The figure shows three views and two pictorial views of one solid part (mm, origin at its lowest corner). Answer the questions. A direction names the side the tool comes from. Coordinates: 2 decimals unless noted, no trailing zeros. Order: outer loops, then holes, each group sorted by start corner. A loop starts at its lowest first (then second) coordinate and runs counter-clockwise, first axis right, second up. Notation, with made-up numbers: M 65,-35 L 99,-35 A20 ccw 99,-2 Z; hole C -17,-16 d4. An arc over 180 degrees is marked long. Use a Markdown table: item, result.
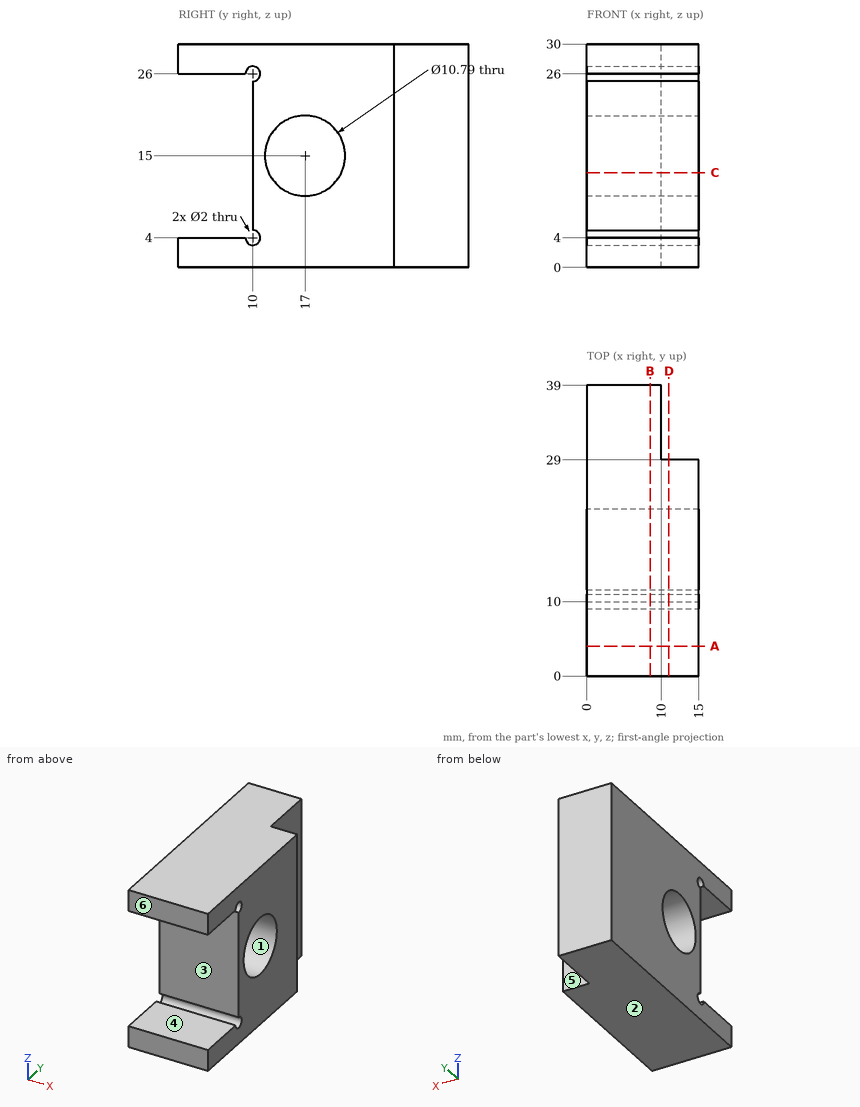
1. Section C-C on z = 12.75 is taken. Determine the outline of the cut face in (x, y).
Answers below:
| item | result |
|---|---|
| outline | M 0,10 L 15,10 L 15,12.1 L 0,12.1 Z; M 0,21.9 L 15,21.9 L 15,29 L 10,29 L 10,39 L 0,39 Z |
2. Find the intervals of material crossed by probe 1 along Z at (x, y) = (4.25, 8.5); probe 2 along Y at (x, z) = (12.5, 28.5); probe 3 along Z at (x, y) = (9.25, 17) (3 decimals), in increasing order.
Answers below:
| item | result |
|---|---|
| probe 1 | 0 to 4, 26 to 30 |
| probe 2 | 0 to 29 |
| probe 3 | 0 to 9.605, 20.395 to 30 |
3. Flat-ended cylindrical pins translate along their axes: P1, Ø1.6, axis at y = 10, z = 4, coming from the +X side; P2, Ø5, axis at x = 12, z = 12.5, coming from the +Y side; P3, Ø2, axis at x = 5, z = 19, coming from the -Y side; P4, Ø5, axis at y = 35, z = 11, coming from the +X side. Find the tip coordinate at first contact, or state that the pin passes through.
Answers below:
| item | result |
|---|---|
| P1 | through |
| P2 | y = 39 |
| P3 | y = 10 |
| P4 | x = 10 |
4. For the marked faces 4, 5 and 6, determine the directions among +Z, -Z, +X, -X, +Y, -Y from which every point of the face is accessible in a straight line to the end or side of a thin tool.
Answers below:
| item | result |
|---|---|
| face 4 | +X, -X, -Y |
| face 5 | +Z, -Z, +X, +Y |
| face 6 | +Z, -Z, +X, -X, -Y |
5. Section A-A on y = 4 is taken. Determine the outline of the cut face in (x, z), then the cut area to 3 significant figures.
Answers below:
| item | result |
|---|---|
| outline | M 0,0 L 15,0 L 15,4 L 0,4 Z; M 0,26 L 15,26 L 15,30 L 0,30 Z |
| area | 120 mm² |
6. For a pull along Y with two mould halves and no side action, classify the marked faces 1, 2 and 3 as +Y half, -Y half, draft (parallel to the pull), parting line (faces both ways), or undercut.
Answers below:
| item | result |
|---|---|
| face 1 | undercut |
| face 2 | draft |
| face 3 | -Y half |
7. Section D-D on x = 11 is taken. Determine the outline of the cut face in (y, z) (3 decimals), then the cut area to 3 significant figures.
Answers below:
| item | result |
|---|---|
| outline | M 0,0 L 29,0 L 29,30 L 0,30 L 0,26 L 9,26 A1 cw long 10,25 L 10,5 A1 cw long 9,4 L 0,4 Z; hole C 17,15 d10.79 |
| area | 554 mm² |
8. Section B-B on x = 8.5 is taken. Determine the outline of the cut face in (y, z) (3 decimals), then the cut area to 3 significant figures.
Answers below:
| item | result |
|---|---|
| outline | M 0,0 L 39,0 L 39,30 L 0,30 L 0,26 L 9,26 A1 cw long 10,25 L 10,5 A1 cw long 9,4 L 0,4 Z; hole C 17,15 d10.79 |
| area | 854 mm² |
